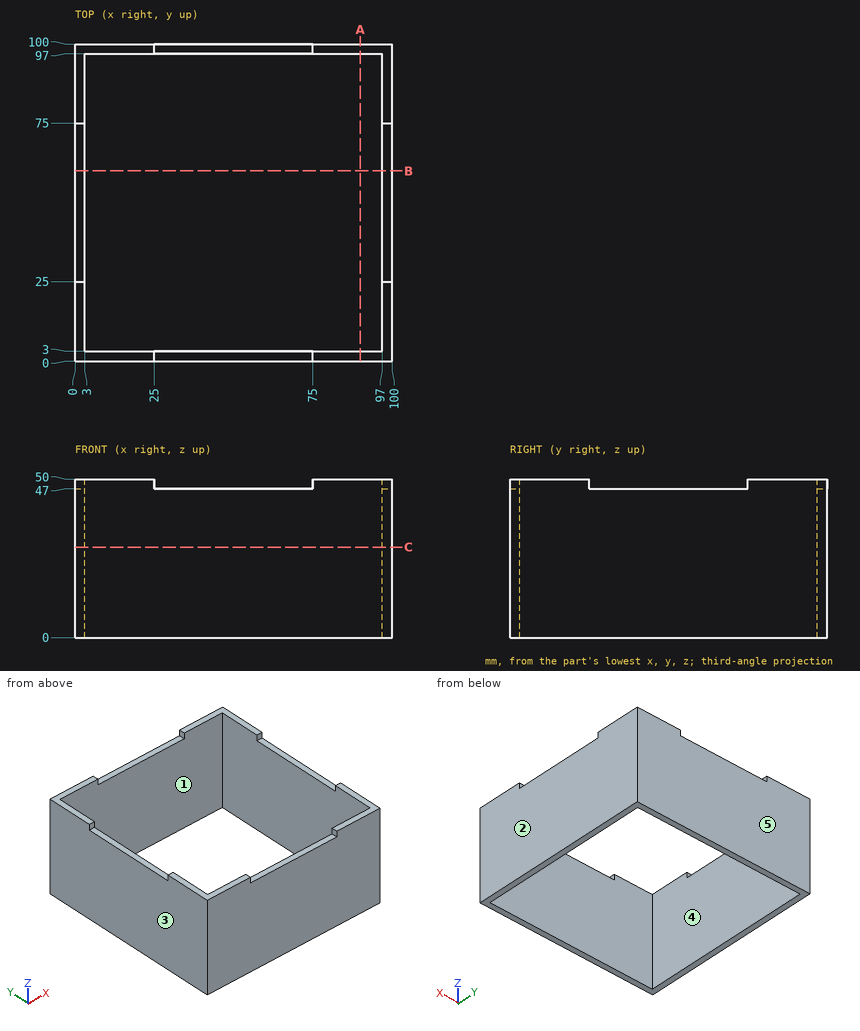
Design review of the part shown in the three views and the two pictorial views. Dimensions are in mm from the part's minimum x, y and z. A direction names the side the tool comes from. Round coordinates to 2 decimals unless told otherwise and drop trailing zeros. Write each loop counter-clockwise with the first axis right and the second up, starting at its lowest first coordinate (ties: lowest second). Pieces come first, ordered by that corner, then holes. Notation, with made-up numbers: (76, 23) - (97, 23) arc R22 ccw to (97, 49) - close; hole circle Ø2 at (-39.75, 44.5). An arc over 180 degrees is marked (long way). Answer as CSV lines item,"result". Start each with the question number.
(1) For pin 1 (2.5 mm diameter, centred on x = 1.5, y = 53, fed in from +Z); pin 2 (1.5 mm diameter, centred on x = 99, z = 48.5, fed in from -Y), all flat-tipped, find the tip position at first contact; note any pin that passes through.
(2) Add section A-A, the plane x = 90. State the section outline as (y, z) points.
(3) Add section C-C, the plane z = 28.5. State the section outline as (x, y) points.
(4) Add section B-B, the plane y = 60. State the section outline as (x, z) points.
(5) For line 1 (X direction, y = 78, z = 27.5), list the stretches that pass through material, from the lowest coordinate up.
(6) Mouldability with a two-part tool opening along Y and no side actions: class the marked faces 3, 4 and 5 as +Y half, -Y half, draft (parallel to the pull), parting line (faces both ways), or undercut.
(7) Machinability: for the marked faces 1 and 2, which of the approach directions +Z, -Z, +X, -X, +Y, -Y give a long, thin tool a straight path to every point of the face, cutting with its end or side? Answer none if there is none.
From the geometry:
1,pin 1,"stops at z = 47"
1,pin 2,"stops at y = 0"
2,outline,"(0, 0) - (3, 0) - (3, 50) - (0, 50) - close; (97, 0) - (100, 0) - (100, 50) - (97, 50) - close"
3,outline,"(0, 0) - (100, 0) - (100, 100) - (0, 100) - close; hole (3, 3) - (97, 3) - (97, 97) - (3, 97) - close"
4,outline,"(0, 0) - (3, 0) - (3, 47) - (0, 47) - close; (97, 0) - (100, 0) - (100, 47) - (97, 47) - close"
5,line 1,"x = 0 to 3, 97 to 100"
6,face 3,"draft"
6,face 4,"undercut"
6,face 5,"+Y half"
7,face 1,"+Z, -Z"
7,face 2,"+Z, -Z, +X, +Y, -Y"
